Autodesk Inventor part; units mm, degrees
ref_plane "YZ Plane" through (0, 0, 0) normal (1, 0, 0) x (0, 1, 0)
ref_plane "XZ Plane" through (0, 0, 0) normal (0, 1, 0) x (-1, 0, 0)
ref_plane "XY Plane" through (0, 0, 0) normal (0, 0, 1) x (1, 0, 0)
sketch "Szkic1" plane through (0, 0, 0) normal (0, 0, 1) x (1, 0, 0)
  circle A0 centre (0, 0) radius 8
  dimension "d0" = 16
extrude "Wyciągnięcie proste1" add sketch "Szkic1" against normal blind 210
sketch "Szkic2" plane through (0, 0, 0) normal (0, 0, 1) x (1, 0, 0)
  line L0 (0, 0) -> (0, 8)
  circle A0 centre (0, 0) radius 8
  circle A1 centre (0, 0) radius 8
  circle A2 centre (0, 0) radius 8
sketch3d "Szkic 3D1"
sketch "Szkic3" plane through (0, 0, 0) normal (0, 0, 1) x (1, 0, 0)
  circle A0 centre (0, 0) radius 8
  circle A1 centre (0, 0) radius 8
  point P0 (0, 8)
sketch3d "Szkic 3D2"
sketch "Szkic4" plane through (0, 0, 0) normal (0, 0, 1) x (1, 0, 0)
  circle A0 centre (0, 0) radius 8
  circle A1 centre (0, 0) radius 8
  point P0 (0, 8)
hole "Otwór1" at (0, 8, -7.5) direction (0, -1, 0) diameter 5 end through all
chamfer "Faza2" distance 2 angle 45 1 edges at (-8, 0, 0)
sketch "Szkic6" plane through (0, 0, -210) normal (0, 0, -1) x (-1, 0, 0)
  point P0 (0, 0)
sketch "Szkic7" plane through (0, 0, -210) normal (0, 0, -1) x (-1, 0, 0)
  circle A0 centre (0, 0) radius 6
extrude "Wyciągnięcie proste2" add sketch "Szkic7" along normal blind 25
sketch "Szkic8" plane through (0, 0, -235) normal (0, 0, -1) x (-1, 0, 0)
  circle A0 centre (0, 0) radius 5
extrude "Wyciągnięcie proste3" add sketch "Szkic8" along normal blind 13
chamfer "Faza3" distance 1 angle 45 1 edges at (5, 0, -248)
CAD build for the part. Positions are in the model's coordinates, mm. A direction names the side the tool comes from. Coordinates: 2 decimals unless noted, no trailing zeros. Order: outer loops, then holes, each group sorted by start corner. A loop starts at its lowest first (then second) coordinate and runs counter-clockwise, first axis right, second up. Notation, with made-up numbers: (66.5, 61) -> (110.5, 61) arc R25 cw to (110.5, 83) -> close; hole circle Ø10 at (-23.5, 0.5). An arc over 180 degrees is marked (long way). Use one line per item in the form item = value. Start each with the question number.
1) Pull direction Z, two halves, no side cores. Call faces 3 (the cylindrical face through (0, 0, -10)), 4 (the cylindrical face through (1.08, 4.88, -240.92)), 5 (the flat face through (0, 0, -248)): +Z half, -Z half, draft (parallel to the pull), parting line (faces both ways), or undercut.
2) Drop flat-ended pins along their axis: pin 1 (3 mm diameter, centred on y = -5, z = -92.5, fed in from +X); pin 2 (3 mm diameter, centred on y = 2.5, z = -180, fed in from -X); pin 3 (1.5 mm diameter, centred on x = -6, z = -140.5, fed in from -Y). Give the stop position or say it passes through.
3) Drill centre lines: L1, parallel to Z at x = -0.25, y = 3.75; L2, parallel to Z at x = 0.5, y = 1.75; L3, parallel to Z at x = 5, y = 1.25. Where is each one in solid material? Low to high. Write a range as [from, to].
4) Band-saw the part on A-A on x = 0. Give the cut face in (y, z).
5) Band-saw the part on C-C on z = -7.5. Give the cut face in (x, y).
6) Tool access for faces 1 (the conical face through (-1.328, 5.979, -0.125)), 2 (the flat face through (-2, 6, -210)): list every direction of +Z, -Z, +X, -X, +Y, -Y with a clear straight run to the whole face (end or side of a thin tool).
7) Band-saw the part on D-D on z = -222. Give the cut face in (x, y), then the cut area to 3 significant figures.
8) Band-saw the part on B-B on y = 0. Give the cut face in (x, z), then the cut area to 3 significant figures.
Entries:
q1.face_3 = undercut
q1.face_4 = draft
q1.face_5 = -Z half
q2.pin_1 = 7.19
q2.pin_2 = -7.94
q2.pin_3 = -6.04
q3.L1 = [-248, -9.99], [-5.01, 0]
q3.L2 = [-248, -9.95], [-5.05, 0]
q3.L3 = [-235, 0]
q4.outline = (-8, -210) -> (-6, -210) -> (-6, -235) -> (-5, -235) -> (-5, -247) -> (-4, -248) -> (4, -248) -> (5, -247) -> (5, -235) -> (6, -235) -> (6, -210) -> (8, -210) -> (8, -10) -> (-8, -10) -> close; (-8, -5) -> (8, -5) -> (8, -2) -> (6, 0) -> (-6, 0) -> (-8, -2) -> close
q5.outline = (-2.5, -7.6) -> (-2.5, 7.6) arc R8 ccw to start; (2.5, -7.6) arc R8 ccw to (2.5, 7.6) -> close
q6.face_1 = +Z
q6.face_2 = -Z
q7.outline = circle Ø12 at (0, 0)
q7.area = 113 mm2
q8.outline = (-8, -210) -> (-6, -210) -> (-6, -235) -> (-5, -235) -> (-5, -247) -> (-4, -248) -> (4, -248) -> (5, -247) -> (5, -235) -> (6, -235) -> (6, -210) -> (8, -210) -> (8, -2) -> (6, 0) -> (-6, 0) -> (-8, -2) -> close; hole circle Ø5 at (0, -7.5)
q8.area = 3,770 mm2
